The figure shows three views and two pictorial views of one solid part (mm, origin at its lowest corner). Answer the questions. Coordinates: 2 decimals unless noted, no trailing zeros. Order: outer loops, then holes, each group sorted by start corner. A loop starts at its lowest first (then second) coordinate and runs counter-clockwise, first axis right, second up. Notation, with made-up numbers: (33, 80) -> (65, 80) arc R30 ccw to (65, 107) -> close; hole circle Ø6 at (-39.5, 67). An arc over 180 degrees is marked (long way). Write item = value, one per line.
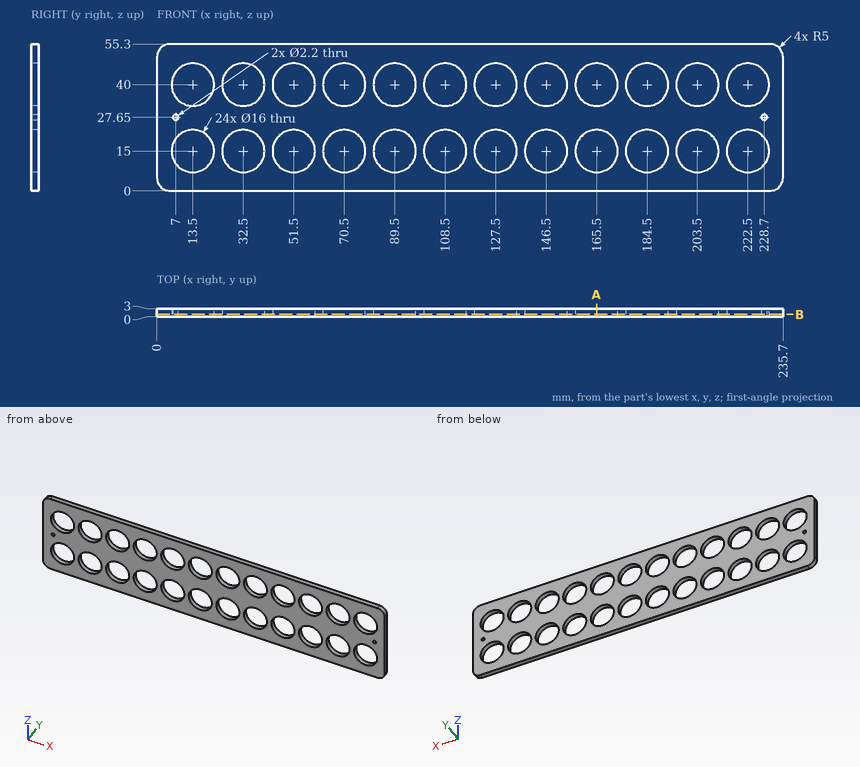
Q1. This flat-tipped pin is pushed along its axis until it touches: pin 1 Ø13 at (x, z) = (13.5, 40) entering from +Y. Where does it stop, or does it pass through?
The answers:
pin_1 = through
Q2. Find the intervals of material crossed by line 1 along Z through (x, y) = (70.5, 1.9); line 2 along Z through (x, y) = (52.5, 0.55), in increasing order.
The answers:
line_1 = 0 to 7, 23 to 32, 48 to 55.3
line_2 = 0 to 7.06, 22.94 to 32.06, 47.94 to 55.3
Q3. Section B-B, the plane y = 0.95 is taken. Give the number of separate pieces and of enclosed holes in the cut face, plus the area to 3 significant figures.
The answers:
separate_pieces = 1
enclosed_holes = 26
area = 8,180 mm2
Q4. Section A-A, the plane x = 165.5 is taken. Give the vertices of the cut face in (y, z), plus the area to 3 significant figures.
The answers:
outline = (0, 0) -> (3, 0) -> (3, 7) -> (0, 7) -> close; (0, 23) -> (3, 23) -> (3, 32) -> (0, 32) -> close; (0, 48) -> (3, 48) -> (3, 55.3) -> (0, 55.3) -> close
area = 69.9 mm2
